from build123d import *

# Parameters (mm, degrees)
F0_W        = 30
F0_H        = 7
F1_DEPTH    = 25
F2_W        = 30
F2_H        = 9
F3_DEPTH    = 7
F4_R        = 2
F5_DEPTH    = 25
F7_DEPTH    = 25
F8_T1_DEPTH = 37.8601958556


# Not quite as in the source:
# - a fillet or chamfer that OpenCascade refuses, or shapes differently, is made with other operations: its cross-section is extruded or revolved along the edge and cut away or added


with BuildPart() as f1:
    # F0 (on Front) → F1 (new body)
    with BuildSketch(Plane.XZ):
        Polygon((-40, 0), (0, 0), (0, 9.8), (-30, 9.8), (-40, 9.8), (-40, 6.8), (-6.3993203272, 6.8), (-6.3993203272, 2), (-40, 2), align=None)
        with Locations((-15, 13.3)):
            Rectangle(F0_W, F0_H)
    extrude(amount=F1_DEPTH)

    # F2 (on face) → F3 (cut)
    with BuildSketch(Plane.XY.offset(16.8)):
        with Locations((-15, -4.5)):
            Rectangle(F2_W, F2_H)
        with Locations((-15, -20.5)):
            Rectangle(F2_W, F2_H)
    extrude(amount=-F3_DEPTH, mode=Mode.SUBTRACT)

    # F4 (on face) → F5 (cut)
    with BuildSketch(Plane.YZ):
        with Locations((-12.5, 13.3)):
            Circle(F4_R)
    extrude(amount=-F5_DEPTH, mode=Mode.SUBTRACT)

    # F6 (on face) → F7 (join)
    with BuildSketch(Plane.YZ):
        Polygon((-16, 16.8), (-25, 9.8), (-16, 9.8), align=None)
        Polygon((0, 9.8), (-9, 16.8), (-9, 9.8), align=None)
    extrude(amount=-F7_DEPTH)

    # F8: chamfer of 6 on 1 edges, made by hand

    # F8_s2 → F8_t1 (cut)
    with BuildSketch(Plane.XZ.offset(-6.4300979278)):
        Polygon((-24, 16.8), (-30, 10.8), (-30, 16.8), align=None)
    extrude(amount=F8_T1_DEPTH, mode=Mode.SUBTRACT)


solid = f1.part
Build history of the part. All positions in model axes, mm. A direction names the side the tool comes from. Give positions to 0.01 mm unless a question says otherwise; leave off trailing zeros. Order: outer loops, then holes, each group sorted by start corner. A loop starts at its lowest first (then second) coordinate and runs counter-clockwise, first axis right, second up. Notation, with made-up numbers: M 34,-6.5 L 71,-6.5 A12 cw 71,9.5 Z; hole C 77,54 d5. An arc over 180 degrees is marked long. Put each result on its own line as item: value.
Item 1: Slice it at A-A, the plane x = -18. Write the cut outline in (y, z), plus the area to 3 significant figures.
From the geometry:
outline: M -25,0 L 0,0 L 0,2 L -25,2 Z; M -25,6.8 L 0,6.8 L 0,9.8 L -9,16.8 L -16,16.8 L -25,9.8 Z; hole C -12.5,13.3 d4
area: 224 mm2
Item 2: Probe line 1 (Z direction, x = -18, y = -12.5); line 2 (Z direction, x = -29.5, y = -13.75); line 3 (Z direction, x = -11, y = -18.75). List the from-to ranges inside material, lowest first. Write a range as [from, to].
From the geometry:
line 1: z = [0, 2], [6.8, 11.3], [15.3, 16.8]
line 2: z = [0, 2], [6.8, 11.3]
line 3: z = [0, 2], [6.8, 14.66]
Item 3: Slice it at D-D, the plane x = -27.5. Write the cut outline in (y, z).
From the geometry:
outline: M -25,0 L 0,0 L 0,2 L -25,2 Z; M -25,6.8 L 0,6.8 L 0,9.8 L -9,9.8 L -9,13.3 L -16,13.3 L -16,9.8 L -25,9.8 Z
Item 4: Slice it at B-B, the plane x = -3.5. Write the cut outline in (y, z).
From the geometry:
outline: M -25,0 L 0,0 L 0,9.8 L -9,16.8 L -16,16.8 L -25,9.8 Z; hole C -12.5,13.3 d4
Item 5: Flat gauge pins, fed straight in: pin 1 Ø2.5 at (x, z) = (-27.5, 13.5) entering from -Y; pin 2 Ø2.5 at (x, z) = (-28.5, 12) entering from +Y; pin 3 Ø6 at (x, y) = (-15.5, -4.5) entering from +Z. Where does each tip first touch, or does it go through?
From the geometry:
pin 1: stops at y = -16
pin 2: stops at y = -9
pin 3: stops at z = 15.63
Item 6: 3-axis set-ups, long thin cutter, end or side, ignore diameter. For faces 1 (the flat face through (-23, -12, 2)), 2 (the cylindrical face through (-12.325, -12.934, 11.348)), 3 (the flat face through (-25, -20, 12)), 4 (the flat face through (-30, -12, 10)), 5 (the flat face through (-27, -9, 12)): which of +Z, -Z, +X, -X, +Y, -Y reach the whole face in a straight line?
From the geometry:
face 1: -X, +Y, -Y
face 2: +X
face 3: +Z, -X, -Y
face 4: +Z, -X, +Y, -Y
face 5: +Z, -X, +Y
Item 7: Slice it at C-C, the plane z = 13.3. Write the cut outline in (x, y).
From the geometry:
outline: M -27.5,-16 L -25,-16 L -25,-20.5 L 0,-20.5 L 0,-14.5 L -25,-14.5 L -25,-10.5 L 0,-10.5 L 0,-4.5 L -25,-4.5 L -25,-9 L -27.5,-9 Z
Item 8: Two-plate mould, pull along Z, no slides. Class faces 6 (the flat face through (-12.325, -20.437, 13.349)), 7 (the flat face through (-6.399, -12, 4)), 8 (the flat face through (-40, -12, 1)), 9 (the flat face through (-23, -12, 6.8)): +Z half, -Z half, draft (parallel to the pull), parting line (faces both ways), or undercut.
From the geometry:
face 6: +Z half
face 7: undercut
face 8: draft
face 9: undercut
